Source: three-view drawing plus pictorial views. Frame: mm from the lowest corner of the part. Coordinates: 2 decimals unless noted, no trailing zeros. Loops run counter-clockwise (first coordinate to the right, second up) from the corner with the lowest first, then second, coordinate; pieces in that order, holes last.
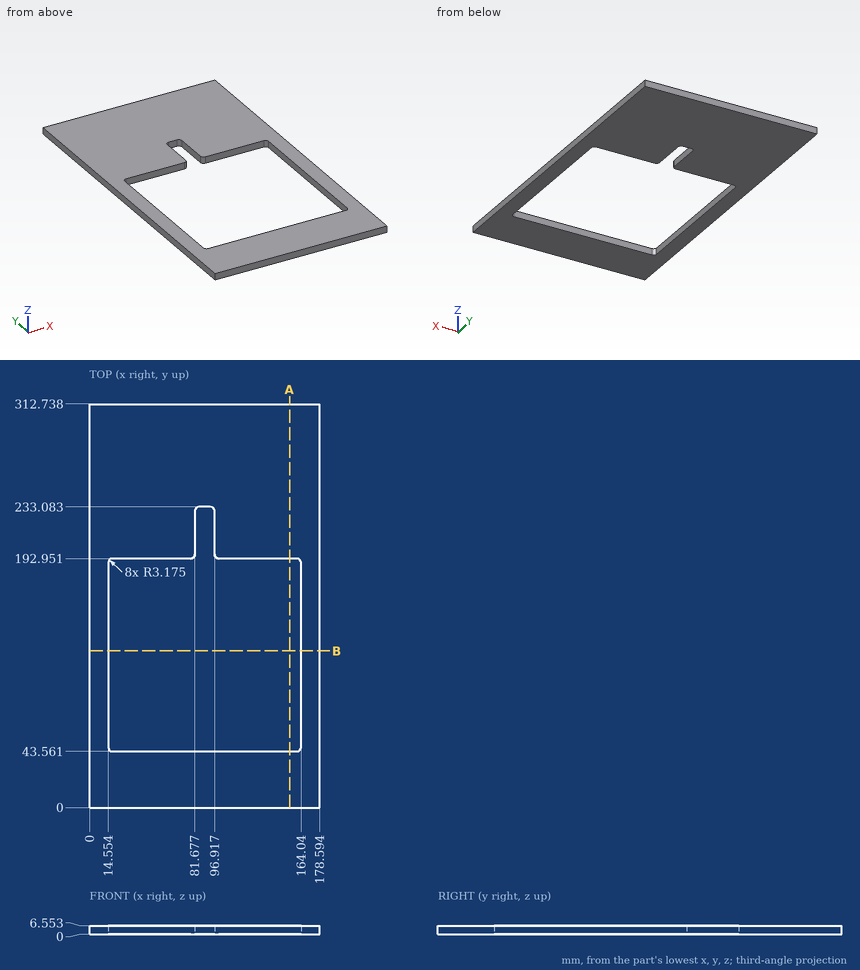
Q1. Section query A-A on x = 155. Return the cut outline in (y, z), then the cut area to 3 significant figures.
Q2. Section query B-B on y = 121.5. Return the cut outline in (x, z) (1 decimal).
Q3. Material intervals for line 1 along Y through (x, z) = (27, 5.25); line 2 along X through (y, z) = (67.5, 3.5) (1 decimal); line 3 along X through (y, z) = (215, 1.25), sorted ascending.
Resolved:
1. outline: (0, 0) - (43.56, 0) - (43.56, 6.55) - (0, 6.55) - close; (192.95, 0) - (312.74, 0) - (312.74, 6.55) - (192.95, 6.55) - close
1. area: 1,070 mm2
2. outline: (0, 0) - (14.6, 0) - (14.6, 6.6) - (0, 6.6) - close; (164, 0) - (178.6, 0) - (178.6, 6.6) - (164, 6.6) - close
3. line 1: y = 0 to 43.56, 192.95 to 312.74
3. line 2: x = 0 to 14.6, 164 to 178.6
3. line 3: x = 0 to 81.68, 96.92 to 178.59
